Autodesk Fusion 360 part; units mm, degrees
sketch "Sketch1" plane through (0, 0, 0) normal (0, 0, 1) x (1, 0, 0)
  line L0 (15, 5) -> (-15, 5)
  line L1 (-15, 5) -> (-15, -5)
  line L2 (-15, -5) -> (15, -5)
  line L3 (15, -5) -> (15, 5)
  line L4 (15, 5) -> (-15, -5) construction
  line L5 (-15, 5) -> (15, -5) construction
  dimension "d1" = 30
  dimension "d2" = 10
extrude "Extrude1" add sketch "Sketch1" along normal blind 10
sketch "Sketch2" plane through (15, 0, 0) normal (1, 0, 0) x (0, 0, -1)
  line L0 (0, -5) -> (0, 5)
  line L1 (0, 5) -> (-10, 5)
  line L2 (-10, 5) -> (-10, -5)
  line L3 (-10, -5) -> (0, -5)
  line L4 (-5, 5) -> (-5, 0) construction
  line L5 (-5, 0) -> (0, 0) construction
  circle A0 centre (-5, 0) radius 1.875
  point P0 (-5, 0)
  dimension "d5" = 3.75
extrude "Extrude2" cut sketch "Sketch2" against normal through all contours A0
sketch "Sketch3" plane through (0, 0, 10) normal (0, 0, 1) x (1, 0, 0)
  line L0 (15, -5) -> (15, 5)
  line L1 (15, 5) -> (-15, 5)
  line L2 (-15, 5) -> (-15, -5)
  line L3 (-15, -5) -> (15, -5)
  line L4 (5, -5) -> (-5, -5)
  line L5 (-5, -5) -> (-5, 5)
  line L6 (-5, 5) -> (5, 5)
  line L7 (5, 5) -> (5, -5)
  line L8 (5, -5) -> (-5, 5) construction
  line L9 (-5, -5) -> (5, 5) construction
  dimension "d7" = 10
extrude "Extrude3" add sketch "Sketch3" along normal blind 10 contours L1 L3 L4 L5 L6 L7
sketch "Sketch4" plane through (0, 0, 20) normal (0, 0, 1) x (1, 0, 0)
  line L0 (5, 5) -> (-5, 5)
  line L1 (-5, 5) -> (-5, -5)
  line L2 (-5, -5) -> (5, -5)
  line L3 (5, -5) -> (5, 5)
  circle A0 centre (0, 0) radius 1.875
  dimension "d10" = 3.75
extrude "Extrude4" cut sketch "Sketch4" along normal up to surface contours A0 end surface at (-5, -0.1867, 3.1343)
hole "Hole1" at (15, 0, 5) direction (-1, 0, 0) diameter 4.5 depth 10 tip angle 118
hole "Hole2" at (-15, 0, 5) direction (1, 0, 0) diameter 4.5 depth 10 tip angle 118
sketch "Sketch5" plane through (0, 0, 20) normal (0, 0, 1) x (1, 0, 0)
  circle A0 centre (0, 0) radius 1.875
  line L0 (5, 5) -> (-5, 5)
  line L1 (-5, 5) -> (-5, -5)
  line L2 (-5, -5) -> (5, -5)
  line L3 (5, -5) -> (5, 5)
  circle A1 centre (0, 0) radius 1.875
hole "Hole3" at (0, 0, 20) direction (0, 0, -1) diameter 4.5 depth 10 tip angle 118
chamfer "Chamfer1" distance 3 angle 45 2 edges at (0, 5, 0) (0, -5, 0)
chamfer "Chamfer1" distance 3 angle 45 10 edges at (-10, -5, 10) (-5, -5, 15) (-5, 0, 10) (-5, 5, 15) (-10, 5, 10) (10, -5, 10) (5, -5, 15) (10, 5, 10) (5, 5, 15) (5, 0, 10)
chamfer "Chamfer2" distance 0.8 angle 45 3 edges at (-15, 2.0977, 5.8136) (15, -2.0977, 5.8136) (-2.0977, 0.8136, 20)
equation "d3 = d2"
equation "d7 = d2"
equation "d8 = d2"
equation "d10 = d5"
equation "d13 = d2"
equation "d16 = d2"
equation "d17 = d14"
equation "d19 = d2"
equation "d20 = d14"
Read the model definition and answer for the solid it produces. Units are mm, in the model's axes. A direction names the side the tool comes from. Round coordinates to 2 decimals unless told otherwise and drop trailing zeros. Write each loop counter-clockwise with the first axis right and the second up, starting at its lowest first coordinate (ties: lowest second). Pieces come first, ordered by that corner, then holes. Notation, with made-up numbers: (11, -5) -> (44, -5) arc R25 ccw to (44, 8) -> close; hole circle Ø11 at (68.5, 22.5). An arc over 180 degrees is marked (long way). Answer in a Markdown table with one row per item. Add a question column.
1) Given P1, Ø2, axis at y = 0, z = 17.5, coming from the +X side; P2, Ø2, axis at x = 0, y = 0, coming from the -Z side; P3, Ø1.2, axis at x = -13, y = 0.5, coming from the +Z side; P4, Ø6, axis at y = 0, z = 5, coming from the +X side, each flat-ended and moving along its own axis, determine where each tip first touches the part or whether it passes through.
2) Which of the six approach directions +Z, -Z, +X, -X, +Y, -Y give full straight-line access (tool end or side, diameter ignored) to faces 1 (the face through (12, 4, 8)), 2 (the face through (11, 0, 10)), 3 (the face through (-4, 3, 16))?
3) Find section A-A, the plane z = 12.25. Determine the outline of the cut face in (x, y), and give its area (3 significant figures).
4) Consider line 1 (Z direction, x = 10.5, y = 0); line 2 (X direction, y = 1.25, z = 14.75); line 3 (Y direction, x = 3.75, z = 5) (3 decimals). Determine where each line is inside the solid, lowest interval first.
5) Find section C-C, the plane x = 12.25. Determine the outline of the cut face in (y, z).
6) Find section B-B, the plane x = 0. Determine the outline of the cut face in (y, z) (3 decimals), and give its area (3 significant figures).
7) Determine the mould class of faces 4 (the face through (4, 3, 17)), 5 (the face through (9.536, -0.676, 2.854)), 6 (the face through (-0.24, 1.86, 7.95)) for opening direction X: pulls with the +X half, pulls with the -X half, needs draft (parallel to the pull), parting line crosses it, or undercut.
8) Find section D-D, the plane y = -4. Determine the outline of the cut face in (x, z).
Findings below:
| question | item | result |
|---|---|---|
| 1 | P1 | x = 5 |
| 1 | P2 | z = 0 |
| 1 | P3 | z = 10 |
| 1 | P4 | x = 14.95 |
| 2 | face 1 | +Z, +X, +Y |
| 2 | face 2 | +Z, +X, +Y, -Y |
| 2 | face 3 | +Z, -X, +Y |
| 3 | outline | (-5.75, -2) -> (-2.75, -5) -> (2.75, -5) -> (5.75, -2) -> (5.75, 2) -> (2.75, 5) -> (-2.75, 5) -> (-5.75, 2) -> close; hole circle Ø4.5 at (0, 0) |
| 3 | area | 81.1 mm² |
| 4 | line 1 | 0 to 2.75, 7.25 to 10 |
| 4 | line 2 | -5 to -1.87, 1.87 to 5 |
| 4 | line 3 | -5 to -1.875, 1.875 to 5 |
| 5 | outline | (-5, 3) -> (-2, 0) -> (2, 0) -> (5, 3) -> (5, 7) -> (2, 10) -> (-2, 10) -> (-5, 7) -> close; hole circle Ø4.5 at (0, 5) |
| 6 | outline | (-5, 3) -> (-2, 0) -> (2, 0) -> (5, 3) -> (5, 20) -> (3.05, 20) -> (2.25, 19.2) -> (2.25, 10) -> (1.875, 9.775) -> (1.875, 5) arc R1.875 cw to (-1.875, 5) -> (-1.875, 9.775) -> (-2.25, 10) -> (-2.25, 19.2) -> (-3.05, 20) -> (-5, 20) -> close |
| 6 | area | 121 mm² |
| 7 | face 4 | pulls with the +X half |
| 7 | face 5 | needs draft |
| 7 | face 6 | undercut |
| 8 | outline | (-15, 2) -> (15, 2) -> (15, 8) -> (8, 8) -> (3, 13) -> (3, 20) -> (-3, 20) -> (-3, 13) -> (-8, 8) -> (-15, 8) -> close |
